Autodesk Inventor part; units mm, degrees
ref_plane "Work Plane1" through (29, 0, 0) normal (0, -1, 0) x (1, 0, 0)
ref_plane "YZ Plane" through (0, 0, 0) normal (1, 0, 0) x (0, 1, 0)
ref_plane "XZ Plane" through (0, 0, 0) normal (0, 1, 0) x (-1, 0, 0)
sketch "Sketch1" plane through (0, 0, 0) normal (0, 0, 1) x (1, 0, 0)
  line L0 (-0.3333, 0) -> (6, 0)
  line L1 (6, 0) -> (6, 1.5)
  line L2 (6, 1.5) -> (3, 1.5)
  line L3 (3, 1.5) -> (2.6932, 1.5)
  line L4 (2.6932, 1.5) -> (0, 1.5)
  line L5 (0, 1.5) -> (0, 2.75)
  line L6 (0, 2.75) -> (-1.7, 2.75)
  line L7 (-1.7, 2.75) -> (-1.7, 1.1547)
  line L8 (-1.7, 1.1547) -> (-1, 1.1547)
  line L9 (-1, 1.1547) -> (-0.3333, 0)
  line L10 (-3.24, 0) -> (7.54, 0)
  line L11 (0, -0.55) -> (0, 3.3)
  line L12 (3, 1.5) -> (0, 1.5) construction
  dimension "d1" = 3
  dimension "d2" = 0.3068
  dimension "d3" = 1.7
  dimension "d4" = 0.7
  dimension "d5" = 60
  dimension "d6" = 3
  dimension "d7" = 3
  dimension "d8" = 2.3094
  dimension "d9" = 5.5
  dimension "d26" = 6
revolve "Body" add sketch "Sketch1" angle 360 about axis through (-0.3333, 0, 0) along (1, 0, 0)
sketch "Sketch2" plane through (-1.7, 0, 0) normal (-1, 0, 0) x (0, 0, 1)
  circle A0 centre (0, 0) radius 1.1547
  line L0 (0, -3.85) -> (0, 3.85)
  line L1 (-3.85, 0) -> (3.85, 0)
  line L2 (1.1547, 0) -> (0.5774, -1)
  line L3 (0.5774, -1) -> (-0.5774, -1)
  line L4 (-0.5774, -1) -> (-1.1547, 0)
  line L5 (-1.1547, 0) -> (-0.5774, 1)
  line L6 (-0.5774, 1) -> (0.5774, 1)
  line L7 (0.5774, 1) -> (1.1547, 0)
extrude "Slot" add sketch "Sketch2" against normal up to next contours L7 A0 | A0 L2 | L6 L0 A0 | A0 L0 L3 | L0 L6 A0 | A0 L3 L0 | L4 A0 | A0 L5
fillet "Fillet1" radius 1 1 edges at (-1.7, -2.75, 0)
chamfer "Chamfer1" distance 0.3067 distance2 0.3067 1 edges at (6, -1.5, 0) measured on face at (6, 0.3952, 0.0397)
ref_plane "Work Plane1" through (29, 0, 0) normal (0, -1, 0) x (1, 0, 0)
fillet "Fillet2" radius 0.1 1 edges at (0, -1.5, 0)
thread "Thread2"
equation "\"d15\" = -0.5 * SPD + 0.5 * GD"
equation "\"d16\" = GUL"
equation "\"GD\" = NND"
equation "\"NLG\" = 6"
equation "\"GEL\" = 4.5"
equation "\"KOD\" = 5.7"
equation "\"KOH\" = 1.65"
equation "\"INTI\" = 1.04"
equation "\"GAL\" = 0.61345 * PTC"
equation "\"GUL\" = 0.61345 * PTC"
equation "\"BDM\" = NND"
equation "\"SW\" = 2"
equation "\"RR\" = 1.45"
equation "\"SPD\" = NND - 1.2269 * PTC"
equation "\"R\" = 0.3"
equation "\"TOA\" = 30deg"
equation "\"GD1\" = THREADDIA - 1.2269 * PTC"
equation "\"THREADDIA\" = 3"
equation "\"PTC\" = 0.5"
equation "\"NND\" = 3"
equation "\"KOH1\" = 0.2"
equation "\"E0\" = 2.303"
properties part number "M3x6 Bolt" material "Stainless Steel"
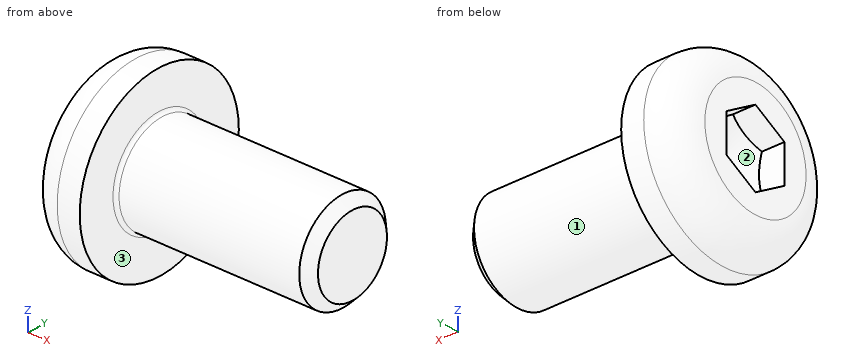
Geometry: final body of the model. Coordinates: model frame, mm. Face numbers are marked on the shaded views. Coordinates: 2 decimals unless noted, no trailing zeros. Loops run counter-clockwise (first coordinate to the right, second up) from the corner with the lowest first, then second, coordinate; pieces in that order, holes last. Notation, with made-up numbers: (29, 60) - (62, 60) arc R5 cw to (62, 67) - close; hole circle Ø7 at (62.25, 72). An arc over 180 degrees is marked (long way). Put each result on its own line as item: value. Start each with the question number.
Q1. Pin query (flat end, axial travel): pin 1 Ø3 at (x, z) = (5, 2) entering from -Y; pin 2 Ø1.5 at (x, z) = (0, 1) entering from +Y; pin 3 Ø3 at (x, y) = (5, 2) entering from +Z. Return the tip coordinate at first contact, or that it passes through.
Q2. Pull-direction query (Y, two-part tool) for the marked faces 1, 2 and 3; classes: released by +Y, released by -Y, zero draft, split by the parting line, or undercut.
Q3. Line query: line 1 (X direction, y = 1.8, z = 0.15); line 2 (Z direction, x = 3.5, y = 1.2); line 3 (Y direction, x = 4.5, z = -0.4). Output: solid intervals per line, ascending.
Q4. Cut plane A-A, the plane x = 5.25. Return loops of the section in (y, z), and give its area (3 significant figures).
Filled sheet:
1. pin 1: y = -1.41
1. pin 2: y = 2.74
1. pin 3: z = 1.41
2. face 1: split by the parting line
2. face 2: undercut
2. face 3: zero draft
3. line 1: -1.7 to 0
3. line 2: -0.9 to 0.9
3. line 3: -1.45 to 1.45
4. outline: circle Ø3 at (0, 0)
4. area: 7.07 mm²
